The model under review builds one solid part; all positions refer to its coordinate system, in mm. A direction names the side the tool comes from. Give positions to 0.01 mm unless a question says otherwise; leave off trailing zeros. Order: outer loops, then holes, each group sorted by start corner. A loop starts at its lowest first (then second) coordinate and runs counter-clockwise, first axis right, second up.
Autodesk Fusion 360 part; units mm, degrees
sketch "Sketch1" plane through (0, 0, 0) normal (0, 0, 1) x (1, 0, 0)
  circle A0 centre (0, 0) radius 25
  dimension "d1" = 50
extrude "Extrude1" add sketch "Sketch1" along normal blind 5
sketch "Sketch2" plane through (0, 0, 5) normal (0, 0, 1) x (-1, 0, 0)
  circle A0 centre (0, 0) radius 25
  circle A1 centre (15, -10) radius 3
  circle A2 centre (-10, -15) radius 3
  circle A3 centre (-15, 10) radius 3
  circle A4 centre (10, 15) radius 3
  dimension "d4" = 6
  dimension "d5" = 6
  dimension "d6" = 6
  dimension "d7" = 6
extrude "Extrude2" cut sketch "Sketch2" against normal blind 5 contours A1 | A2 | A3 | A4
sketch "Sketch3" plane through (0, 0, 5) normal (0, 0, 1) x (-1, 0, 0)
  circle A0 centre (-10, -15) radius 3
  circle A1 centre (-15, 10) radius 3
  circle A2 centre (15, -10) radius 3
  circle A3 centre (10, 15) radius 3
  circle A4 centre (0, 0) radius 25
  circle A5 centre (15, -10) radius 5
  circle A6 centre (-10, -15) radius 5
  circle A7 centre (-15, 10) radius 5
  circle A8 centre (10, 15) radius 5
  dimension "d10" = 10
  dimension "d11" = 10
  dimension "d12" = 10
  dimension "d13" = 10
extrude "Extrude3" cut sketch "Sketch3" against normal blind 2 contours A5 | A6 | A7 | A8
sketch "Sketch4" plane through (0, 0, 5) normal (0, 0, 1) x (-1, 0, 0)
  circle A0 centre (-10, -15) radius 5
  circle A1 centre (-15, 10) radius 5
  circle A2 centre (15, -10) radius 5
  circle A3 centre (10, 15) radius 5
  circle A4 centre (0, 0) radius 25
  circle A5 centre (0, 0) radius 2.375
  dimension "d16" = 4.75
extrude "Extrude4" cut sketch "Sketch4" against normal blind 21 contours A5
sketch "Sketch7" plane through (0, 0, 0) normal (0, 0, -1) x (1, 0, 0)
  circle A0 centre (0, 0) radius 2.375
  circle A1 centre (10, -15) radius 3
  circle A2 centre (15, 10) radius 3
  circle A3 centre (-15, -10) radius 3
  circle A4 centre (-10, 15) radius 3
  circle A5 centre (0, 0) radius 25
  circle A6 centre (0, 0) radius 4.875
  dimension "d22" = 9.75
extrude "Extrude6" add sketch "Sketch7" along normal blind 5 contours A6
Item 1: Take a section at A-A (x = 0). Give the boundary of the cut face in (y, z) (3 decimals).
Values found:
outline: (-25, 0) - (-4.875, 0) - (-4.875, -5) - (-2.375, -5) - (-2.375, 5) - (-25, 5) - close; (2.375, -5) - (4.875, -5) - (4.875, 0) - (25, 0) - (25, 5) - (2.375, 5) - close
Item 2: Clearance check with flat-ended pins moving along their axes: pin 1 Ø8 at (x, y) = (12.5, -11.5) entering from +Z; pin 2 Ø8 at (x, y) = (15, -10) entering from +Z; pin 3 Ø3.5 at (x, y) = (-15, 10) entering from -Z; pin 4 Ø4 at (x, y) = (16.5, 9) entering from -Z. State where each tip first meets the part, or that it passes through.
Values found:
pin 1: stops at z = 5
pin 2: stops at z = 3
pin 3: passes through
pin 4: stops at z = 0
Item 3: Take a section at D-D (x = 19). Give the boundary of the cut face in (y, z), and give its area (3 significant figures).
Values found:
outline: (-16.25, 0) - (16.25, 0) - (16.25, 5) - (-7, 5) - (-7, 3) - (-13, 3) - (-13, 5) - (-16.25, 5) - close
area: 150 mm2
Item 4: Take a section at C-C (z = -2). Give the boundary of the cut face in (x, y) (3 decimals), and give its area (3 significant figures).
Values found:
outline: circle Ø9.75 at (0, 0); hole circle Ø4.75 at (0, 0)
area: 56.9 mm2
Item 5: For line 1 (Y direction, x = -15, z = 1.2); line 2 (Z direction, x = -11.5, y = -2); line 3 (Y direction, x = -11.5, z = 3.75), list the stretches that pass through material, from the lowest coordinate up.
Values found:
line 1: y = -20 to 7, 13 to 20
line 2: z = 0 to 5
line 3: y = -22.2 to -19.77, -10.23 to 6.43, 13.57 to 22.2
Item 6: Take a section at B-B (y = -8.5). Give the boundary of the cut face in (x, z).
Values found:
outline: (-23.51, 0) - (12.4, 0) - (12.4, 3) - (10.23, 3) - (10.23, 5) - (-23.51, 5) - close; (17.6, 0) - (23.51, 0) - (23.51, 5) - (19.77, 5) - (19.77, 3) - (17.6, 3) - close
Item 7: For faces 1 (the cylindrical face through (23.846, -7.509, 2.465)), 2 (the cylindrical face through (-12.307, -10.564, 4.014)), list the 3-axis set-ups (+Z, -Z, +X, -X, +Y, -Y) from which the entire face can be reached by the end or side of a thin tool; tool diameter is ignored.
Values found:
face 1: +Z, -Z
face 2: +Z
Item 8: Draft analysis for pull direction X (two halves, no side actions). For faces 3 (the cylindrical face through (-0.635, 4.834, -2.465)), 4 (the cylindrical face through (19, -13, 4)), 5 (the flat face through (-0.3, -5.2, 0)), state which applies: released by +X, released by -X, zero draft, split by the parting line, or undercut.
Values found:
face 3: split by the parting line
face 4: undercut
face 5: zero draft
